Can you work these out from the model? Positions are in its coordinate system, mm. Face numbers are marked on the shaded views. Round coordinates to 2 decimals unless told otherwise and drop trailing zeros. Loops run counter-clockwise (first coordinate to the right, second up) from the corner with the lowest first, then second, coordinate; pieces in that order, holes last. Notation, with made-up numbers: (6, 47.5) -> (43, 47.5) arc R11 ccw to (43, 61.5) -> close; hole circle Ø10 at (16, 44). An arc over 180 degrees is marked (long way). Write item = value, one per line.
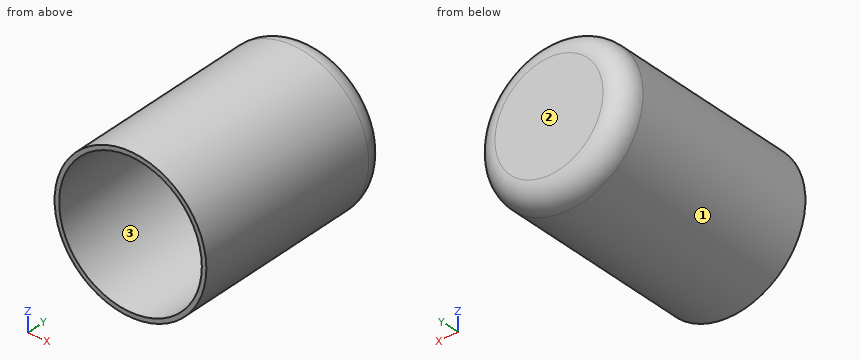
from build123d import *

# Parameters (mm, degrees)
F0_R     = 42.594898
F1_DEPTH = 121.92
F2_R     = 12.264205
F3_T     = -2.54


with BuildPart() as f1:
    # F0 (on Front) → F1 (new body)
    with BuildSketch(Plane.XZ):
        Circle(F0_R)
    extrude(amount=-F1_DEPTH)

    # F2
    f2_edges = [f1.edges().sort_by_distance(p)[0] for p in [
        (-42.594898, 121.92, 0),
    ]]
    fillet(f2_edges, radius=F2_R)

    # F3
    f3_openings = [f1.faces().sort_by_distance(p)[0] for p in [
        (0, 0, 0),
    ]]
    offset(amount=F3_T, openings=f3_openings)


solid = f1.part
1. We'd pull the mould along Z, two halves only. Please class the marked faces 1, 2 and 3: released by +Z, released by -Z, zero draft, split by the parting line, or undercut.
Entries:
face_1 = split by the parting line
face_2 = zero draft
face_3 = undercut
2. I'm going to push flat-ended pins straight in: pin 1 (1 mm diameter, centred on x = -28, y = 54, fed in from +Z); pin 2 (6 mm diameter, centred on y = 21, z = -22, fed in from -X); pin 3 (4 mm diameter, centred on x = 16.5, y = 29, fed in from -Z). Where does each tip first touch, or does it pass through?
Entries:
pin_1 = 32.53
pin_2 = -38.12
pin_3 = -40.05
3. Suppose I cut it at B-B, the plane z = 0. List the corners of the cut face in (x, y) for me, and give its area (3 significant figures).
Entries:
outline = (-42.59, 0) -> (-40.05, 0) -> (-40.05, 109.66) arc R9.72 cw to (-30.33, 119.38) -> (30.33, 119.38) arc R9.72 cw to (40.05, 109.66) -> (40.05, 0) -> (42.59, 0) -> (42.59, 109.66) arc R12.26 ccw to (30.33, 121.92) -> (-30.33, 121.92) arc R12.26 ccw to (-42.59, 109.66) -> close
area = 799 mm²
4. I need wall thicknesses on line 1 (Z direction, x = 0, y = 62); line 2 (X direction, y = 49.5, z = -1); line 3 (X direction, y = 69.5, z = 19.5). Which ranges of each line are inside material? Lowest first, please. Write a range as [from, to].
Entries:
line_1 = [-42.59, -40.05], [40.05, 42.59]
line_2 = [-42.58, -40.04], [40.04, 42.58]
line_3 = [-37.87, -34.99], [34.99, 37.87]
5. Suppose I cut it at C-C, the plane y = 68. List the corners of the cut face in (x, z) for me, and give its area (3 significant figures).
Entries:
outline = circle Ø85.19 at (0, 0); hole circle Ø80.11 at (0, 0)
area = 660 mm²
6. Suppose I cut it at A-A, the plane x = 0. List the corners of the cut face in (y, z) for me.
Entries:
outline = (0, -42.59) -> (109.66, -42.59) arc R12.26 ccw to (121.92, -30.33) -> (121.92, 30.33) arc R12.26 ccw to (109.66, 42.59) -> (0, 42.59) -> (0, 40.05) -> (109.66, 40.05) arc R9.72 cw to (119.38, 30.33) -> (119.38, -30.33) arc R9.72 cw to (109.66, -40.05) -> (0, -40.05) -> close
